```python
from build123d import *

# Parameters (mm, degrees)
F0_W     = 20.32
F0_H     = 20.32
F1_DEPTH = 2.54
F0_W_2   = 25.4
F0_H_2   = 25.4
F2_DEPTH = 21.59
F3_W     = 20.32
F3_H     = 20.32
F4_DEPTH = 0.635


with BuildPart() as f1:
    # F0 (on Top) → F1 (new body)
    with BuildSketch(Plane.XY):
        Rectangle(F0_W, F0_H)
    extrude(amount=F1_DEPTH)

    # F0 (on Top) → F2 (join)
    with BuildSketch(Plane.XY):
        Rectangle(F0_W_2, F0_H_2)
        Rectangle(F0_W, F0_H, mode=Mode.SUBTRACT)
    extrude(amount=F2_DEPTH)

    # F3 (on face) → F4 (join)
    with BuildSketch(Plane.XY.offset(21.59)):
        Polygon((-11.991714, 11.43), (-11.229714, 11.43), (-11.229714, -11.43), (-11.229714, -12.7), (11.030424, -12.7), (11.030424, -11.454967), (11.030424, 11.405033), (11.792424, 11.405033), (11.792424, -11.454967), (11.792424, -12.7), (12.7, -12.7), (12.7, 12.7), (-12.7, 12.7), (-12.7, -12.7), (-11.991714, -12.7), (-11.991714, -11.43), align=None)
        Rectangle(F3_W, F3_H, mode=Mode.SUBTRACT)
    extrude(amount=F4_DEPTH)


solid = f1.part
```
Part model, mm, in its own coordinate system. A direction names the side the tool comes from. Coordinates: 2 decimals unless noted, no trailing zeros. Loops run counter-clockwise (first coordinate to the right, second up) from the corner with the lowest first, then second, coordinate; pieces in that order, holes last. Notation, with made-up numbers: (58, -40) - (106, -40) arc R25 cw to (106, -9) - close; hole circle Ø7 at (31, 79.25). An arc over 180 degrees is marked (long way). Write item = value, one per line. Start each with the question number.
Item 1: 3-axis set-ups, long thin cutter, end or side, ignore diameter. For faces 5 (the flat face through (-10.16, 0, 12)), 6 (the flat face through (0, -12.7, 11)): which of +Z, -Z, +X, -X, +Y, -Y reach the whole face in a straight line?
Item 2: Cut at A-A, the plane z = 15.75. Give the cut face in (x, y), and give its area (3 significant figures).
Item 3: Cut at C-C, the plane x = -1.5. Give the cut face in (y, z) (3 decimals).
Item 4: Wall check: L1, parallel to X at y = 7.25, z = 21; L2, parallel to Z at x = 6.25, y = -10. Give the ranges that are in metal, low to high. Write a range as from..to.
Item 5: Mould opens along X. For faces 1 (the flat face through (12.7, 0, 11)), 2 (the flat face through (0, 0, 2.54)), 3 (the flat face through (0, 12.7, 11)), 4 (the flat face through (10.16, 0, 12)) say: released by +X, released by -X, zero draft, split by the parting line, or undercut.
Item 6: Cut at B-B, the plane y = -6.75. Give the cut face in (x, z) (3 decimals), and give its area (3 significant figures).
Item 7: Flat gauge pin, fed straight in: pin 1 Ø10 at (x, y) = (-3.5, -2.5) entering from +Z. Where does the tip first touch, or does it go through?
The answers:
q1.face_5 = +Z
q1.face_6 = +Z, -Z, +X, -X, -Y
q2.outline = (-12.7, -12.7) - (12.7, -12.7) - (12.7, 12.7) - (-12.7, 12.7) - close; hole (-10.16, -10.16) - (10.16, -10.16) - (10.16, 10.16) - (-10.16, 10.16) - close
q2.area = 232 mm2
q3.outline = (-12.7, 0) - (12.7, 0) - (12.7, 22.225) - (10.16, 22.225) - (10.16, 2.54) - (-10.16, 2.54) - (-10.16, 22.225) - (-12.7, 22.225) - close
q4.L1 = -12.7..-10.16, 10.16..12.7
q4.L2 = 0..2.54
q5.face_1 = released by +X
q5.face_2 = undercut
q5.face_3 = zero draft
q5.face_4 = undercut
q6.outline = (-12.7, 0) - (12.7, 0) - (12.7, 22.225) - (11.792, 22.225) - (11.792, 21.59) - (11.03, 21.59) - (11.03, 22.225) - (10.16, 22.225) - (10.16, 2.54) - (-10.16, 2.54) - (-10.16, 22.225) - (-11.23, 22.225) - (-11.23, 21.59) - (-11.992, 21.59) - (-11.992, 22.225) - (-12.7, 22.225) - close
q6.area = 164 mm2
q7.pin_1 = 2.54
